```python
from build123d import *

# Parameters (mm, degrees)
F0_W        = 600
F0_H        = 500
F1_DEPTH    = 800
F2_W        = 500
F2_H        = 80
F3_DEPTH    = 25
F5_DEPTH    = 50
F6_T1_DEPTH = 145.0048285071
F6_T4_ANGLE = 180
F6_T6_ANGLE = 180
F7_W        = 40
F7_H        = 110
F8_DEPTH    = 25
F9_R        = 4.99999
F10_W       = 630
F10_H       = 500
F11_DEPTH   = 25
F12_DEPTH   = 600
F13_W       = 600
F13_H       = 800
F14_DEPTH   = 500
F15_W       = 630
F15_H       = 25
F16_DEPTH   = 470
F17_W       = 500
F17_H       = 80
F18_DEPTH   = 25
F19_W       = 575
F19_H       = 80
F20_DEPTH   = 25


# Not quite as in the source:
# - a fillet or chamfer that OpenCascade refuses, or shapes differently, is made with other operations: its cross-section is extruded or revolved along the edge and cut away or added
# - a fillet or chamfer is up to 0.001 mm smaller than in the source, because OpenCascade refuses the exact size


with BuildPart() as f1:
    # F0 (on Top) → F1 (new body)
    with BuildSketch(Plane.XY):
        Rectangle(F0_W, F0_H)
    extrude(amount=F1_DEPTH)

    # F2 (on face) → F3 (cut)
    with BuildSketch(Plane.YZ.offset(300)):
        with Locations((0, 40)):
            Rectangle(F2_W, F2_H)
    extrude(amount=-F3_DEPTH, mode=Mode.SUBTRACT)

    # F4 (on face) → F5 (join)
    with BuildSketch(Plane.YZ.offset(300)):
        with BuildLine():
            ThreePointArc((-220, 750), (-223.5355339059, 748.5355339059), (-225, 745))
            Line((-225, 745), (-225, 625))
            ThreePointArc((-225, 625), (-223.5355339059, 621.4644660941), (-220, 620))
            ThreePointArc((-220, 620), (-216.4644660941, 621.4644660941), (-215, 625))
            Line((-215, 625), (-215, 745))
            ThreePointArc((-215, 745), (-216.4644660941, 748.5355339059), (-220, 750))
        make_face()
    extrude(amount=F5_DEPTH)

    # F6: fillet of radius 5 on 4 edges, made by hand

    # F6_s2 → F6_t1 (cut)
    with BuildSketch(Plane.XY.offset(612.4975857464)):
        with BuildLine():
            ThreePointArc((344.9990343146, -225.0004), (348.5355339059, -223.5355339059), (350.0004, -219.9990343146))
            Line((350.0004, -219.9990343146), (350.5005365685, -219.9990343146))
            ThreePointArc((350.5005365685, -219.9990343146), (350.5001365685, -222.4995171573), (350.5001365685, -225))
            Line((350.5001365685, -225), (350, -225.5001365685))
            ThreePointArc((350, -225.5001365685), (347.4995171573, -225.5001365685), (344.9990343146, -225.5005365685))
            Line((344.9990343146, -225.5005365685), (344.9990343146, -225.0004))
        make_face()
        with BuildLine():
            ThreePointArc((344.9990343146, -214.9996), (348.5355339059, -216.4644660941), (350.0004, -220.0009656854))
            Line((350.0004, -220.0009656854), (350.5005365685, -220.0009656854))
            ThreePointArc((350.5005365685, -220.0009656854), (350.5001365685, -217.5004828427), (350.5001365685, -215))
            Line((350.5001365685, -215), (350, -214.4998634315))
            ThreePointArc((350, -214.4998634315), (347.4995171573, -214.4998634315), (344.9990343146, -214.4994634315))
            Line((344.9990343146, -214.4994634315), (344.9990343146, -214.9996))
        make_face()
    extrude(amount=F6_T1_DEPTH, mode=Mode.SUBTRACT)

    # F6_s3 → F6_t4 (revolve, cut)
    with BuildSketch(Plane.XY.offset(745)):
        with BuildLine():
            ThreePointArc((344.9990343146, -225.0004), (348.5351924681, -223.5358753108), (350.0003999068, -220))
            Line((350.0003999068, -220), (350.5005364913, -220))
            Line((350.5005364913, -220), (350.5001365685, -225))
            Line((350.5001365685, -225), (350, -225.5001365685))
            ThreePointArc((350, -225.5001365685), (347.4995171573, -225.5001365685), (344.9990343146, -225.5005365685))
            Line((344.9990343146, -225.5005365685), (344.9990343146, -225.0004))
        make_face()
    revolve(axis=Axis((350, -220, 745), (-1, 0, 0)), revolution_arc=F6_T4_ANGLE, mode=Mode.SUBTRACT)

    # F6_s5 → F6_t6 (revolve, cut)
    with BuildSketch(Plane.XY.offset(625)):
        with BuildLine():
            ThreePointArc((344.9990343146, -214.9996), (348.5351924681, -216.4641246892), (350.0003999068, -220))
            Line((350.0003999068, -220), (350.5005364913, -220))
            Line((350.5005364913, -220), (350.5001365685, -215))
            Line((350.5001365685, -215), (350, -214.4998634315))
            ThreePointArc((350, -214.4998634315), (347.4995171573, -214.4998634315), (344.9990343146, -214.4994634315))
            Line((344.9990343146, -214.4994634315), (344.9990343146, -214.9996))
        make_face()
    revolve(axis=Axis((350, -220, 625), (-1, 0, 0)), revolution_arc=F6_T6_ANGLE, mode=Mode.SUBTRACT)

    # F7 (on face) → F8 (cut)
    with BuildSketch(Plane(origin=(0, -215, 0), x_dir=(-1, 0, 0), z_dir=(0, 1, 0))):
        with Locations((-320, 685)):
            Rectangle(F7_W, F7_H)
    extrude(amount=-F8_DEPTH, mode=Mode.SUBTRACT)

    # F9 (radius 5 in the source; OpenCascade refuses exactly that, so slightly less here)
    f9_edges = [f1.edges().sort_by_distance(p)[0] for p in [
        (320, -215, 740),
        (340, -215, 685),
        (320, -215, 630),
        (320, -225, 740),
        (340, -225, 685),
        (320, -225, 630),
    ]]
    fillet(f9_edges, radius=F9_R)

    # F10 (on face) → F11 (join)
    with BuildSketch(Plane.XY.offset(800)):
        with Locations((15, 0)):
            Rectangle(F10_W, F10_H)
    extrude(amount=F11_DEPTH)

    # F12 (add): a face of the model
    f12_faces = [f1.faces().sort_by_distance(p)[0] for p in [
        (-0.6860759494, 250, 414.6164556962),
    ]]
    extrude(f12_faces, amount=F12_DEPTH)

    # F13 (on face) → F14 (join)
    with BuildSketch(Plane.YZ.offset(300)):
        with Locations((550, 400)):
            Rectangle(F13_W, F13_H)
    extrude(amount=F14_DEPTH)

    # F15 (on face) → F16 (join)
    with BuildSketch(Plane.YZ.offset(330)):
        with Locations((535, 812.5)):
            Rectangle(F15_W, F15_H)
    extrude(amount=F16_DEPTH)

    # F17 (on face) → F18 (cut)
    with BuildSketch(Plane.XZ.offset(-250)):
        with Locations((550, 40)):
            Rectangle(F17_W, F17_H)
    extrude(amount=-F18_DEPTH, mode=Mode.SUBTRACT)

    # F19 (on face) → F20 (join)
    with BuildSketch(Plane(origin=(300, 0, 0), x_dir=(0, -1, 0), z_dir=(-1, 0, 0))):
        with Locations((-562.5, 40)):
            Rectangle(F19_W, F19_H)
    extrude(amount=F20_DEPTH)


solid = f1.part
```
Source: CAD feature listing. Evaluate the final solid. Frame: model axes, mm. A direction names the side the tool comes from. Coordinates: 2 decimals unless noted, no trailing zeros. Write each loop counter-clockwise with the first axis right and the second up, starting at its lowest first coordinate (ties: lowest second). Pieces come first, ordered by that corner, then holes. Notation, with made-up numbers: (57, 12.25) -> (111, 12.25) arc R6 ccw to (111, 19.25) -> close; hole circle Ø5 at (26.25, 87.5). An arc over 180 degrees is marked (long way). Return JSON: item names as keys, results as strings. Group by question number.
1) Ray query, line 1 along Y through (x, z) = (457.5, 763.5); line 2 along X through (y, z) = (151, 561.5). Return the intervals inside material, ascending.
2) Contact query for a flat-ended pin moving along its axis: P1, Ø22.5, axis at x = 328.5, z = 680.5, coming from the -Y side. Output: stop coordinate, or through.
3) Section query B-B, the plane x = 368.5. Return loops of the section in (y, z), plus the area to 3 significant figures.
4) Section query A-A, the plane y = 47.5. Return loops of the section in (x, z).
5) Section query C-C, the plane z = 180.5. Return loops of the section in (x, y).
6) Set-up query: faces 1 (the face through (120, 415, 825)), 2 (the face through (275, 9, 39)). Return all of +Z, -Z, +X, -X, +Y, -Y with unobstructed straight access to the full face (end or side cutting, diameter ignored); none if empty.
From the geometry:
{
 "1": {"line 1": "250 to 850", "line 2": "-300 to 300"},
 "2": {"P1": "y = 250"},
 "3": {"outline": "(220, 800) -> (250, 800) -> (250, 80) -> (275, 80) -> (275, 0) -> (850, 0) -> (850, 825) -> (220, 825) -> close", "area": "494,000 mm²"},
 "4": {"outline": "(-300, 0) -> (275, 0) -> (275, 80) -> (300, 80) -> (300, 800) -> (330, 800) -> (330, 825) -> (-300, 825) -> close"},
 "5": {"outline": "(-300, -250) -> (300, -250) -> (300, 250) -> (800, 250) -> (800, 850) -> (-300, 850) -> close"},
 "6": {"face 1": "+Z, +X, -X, +Y, -Y", "face 2": "-Z, +X, -Y"}
}
